```python
from build123d import *

# Parameters (mm, degrees)
BOSS_EXTRUDE1_DEPTH = 178
SKETCH2_W           = 150
SKETCH2_H           = 168
CUT_EXTRUDE1_DEPTH  = 33


with BuildPart() as part:
    # Sketch1 → Boss-Extrude1 (new body)
    with BuildSketch(Plane.XY):
        Polygon((169, -9), (9, -9), (9, 0), (0, 0), (0, 20), (9, 20), (9, 29), (169, 29), (169, 20), (178, 20), (178, 0), (169, 0), align=None)
    extrude(amount=-BOSS_EXTRUDE1_DEPTH)

    # Sketch2 → Cut-Extrude1 (cut)
    with BuildSketch(Plane(origin=(0, 29, 0), x_dir=(1, 0, 0), z_dir=(0, 1, 0))):
        with Locations((89, 89)):
            Rectangle(SKETCH2_W, SKETCH2_H)
    extrude(amount=-CUT_EXTRUDE1_DEPTH, mode=Mode.SUBTRACT)


solid = part.part
```
Geometry check sheet. Reference: the model listing, model coordinates, mm. A direction names the side the tool comes from. Coordinates: 2 decimals unless noted, no trailing zeros. Order: outer loops, then holes, each group sorted by start corner. A loop starts at its lowest first (then second) coordinate and runs counter-clockwise, first axis right, second up. Notation, with made-up numbers: (-25, 66) - (33, 66) arc R28 ccw to (33, 93) - close; hole circle Ø1 at (68.25, 83). An arc over 180 degrees is marked (long way). Answer as a JSON object with one key per item and string values. Group by question number.
Item 1: Draft check along X on faces 1 (the face through (169, -4, -88)), 2 (the face through (174, 0, -88)), 3 (the face through (88, -4, -90)). Enter one of: +X half, -X half, draft (parallel to the pull), parting line (faces both ways), or undercut.
Item 2: Scan lines: probe 1 along Z at (x, y) = (74, 6); probe 2 along X at (y, z) = (13, -142.5); probe 3 along X at (y, z) = (-1, -27.5). Record each from-to range of solid material in increasing order.
Item 3: Sectioned sample at A-A, the plane y = 12.5. Record the cut outline in (x, z), and give its area (3 significant figures).
Item 4: Depth check by flat-ended pin: pin 1 Ø2.5 at (x, z) = (171.5, -83.5) entering from +Y; pin 2 Ø2.5 at (x, z) = (171.5, -108) entering from -Y; pin 3 Ø7 at (y, z) = (26.5, -125) entering from +X. Enter the tip coordinate at first touch or a pass-through.
Item 5: Tool access check on faces 4 (the face through (9, 24, -88)), 5 (the face through (88, 13, -173)), 6 (the face through (90, 10, -178)), 7 (the face through (9, -5, -88)), 8 (the face through (173, 20, -88)). Record the directions out of +Z, -Z, +X, -X, +Y, -Y that give a thin tool (end or side, any length) a straight path to the whole face; none if there is none.
Item 6: Sectioned sample at C-C, the plane x = 86. Record the cut outline in (y, z), and give its area (3 significant figures).
Item 7: Sectioned sample at B-B, the plane z = -132.5. Record the cut outline in (x, y), and give its area (3 significant figures).
Resolved:
{
 "1": {"face 1": "+X half", "face 2": "draft", "face 3": "undercut"},
 "2": {"probe 1": "-178 to -173, -5 to 0", "probe 2": "0 to 14, 164 to 178", "probe 3": "9 to 14, 164 to 169"},
 "3": {"outline": "(0, -178) - (178, -178) - (178, 0) - (0, 0) - close; hole (14, -173) - (164, -173) - (164, -5) - (14, -5) - close", "area": "6,480 mm^2"},
 "4": {"pin 1": "y = 20", "pin 2": "y = 0", "pin 3": "x = 169"},
 "5": {"face 4": "+Z, -Z, -X, +Y", "face 5": "+Y", "face 6": "-Z, +X, -X, +Y, -Y", "face 7": "+Z, -Z, -X, -Y", "face 8": "+Z, -Z, +X, +Y"},
 "6": {"outline": "(-9, -178) - (29, -178) - (29, -173) - (-4, -173) - (-4, -5) - (29, -5) - (29, 0) - (-9, 0) - close", "area": "1,220 mm^2"},
 "7": {"outline": "(0, 0) - (9, 0) - (9, -9) - (169, -9) - (169, 0) - (178, 0) - (178, 20) - (169, 20) - (169, 29) - (164, 29) - (164, -4) - (14, -4) - (14, 29) - (9, 29) - (9, 20) - (0, 20) - close", "area": "1,490 mm^2"}
}
